The model under review builds one solid part; all positions refer to its coordinate system, in mm. Face numbers are marked on the shaded views. Give positions to 0.01 mm unless a question says otherwise; leave off trailing zeros. Order: outer loops, then holes, each group sorted by start corner. A loop starts at its lowest first (then second) coordinate and runs counter-clockwise, first axis right, second up. Notation, with made-up numbers: (-2.75, -8) - (4.25, -8) arc R31 cw to (4.25, 20) - close; hole circle Ø5 at (75.25, -6.5). An arc over 180 degrees is marked (long way). Put each result on its own line as item: value.
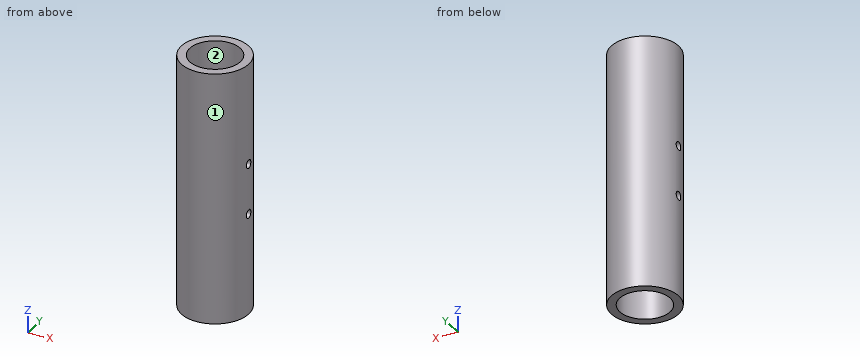
```python
from build123d import *

# Parameters (mm, degrees)
SKETCH1_R               = 20
BOSS_EXTRUDE1_DEPTH     = 150
SKETCH2_R               = 15
CUT_EXTRUDE1_DEPTH      = 150
CUT_EXTRUDE2_DEPTH      = 153.643375225
CUT_EXTRUDE2_DEPTH_BACK = 153.643375225
SKETCH3_R               = 2.5


with BuildPart() as part:
    # Sketch1 → Boss-Extrude1 (new body)
    with BuildSketch(Plane.XY):
        Circle(SKETCH1_R)
    extrude(amount=BOSS_EXTRUDE1_DEPTH)

    # Sketch2 → Cut-Extrude1 (cut)
    with BuildSketch(Plane.XY.offset(150)):
        Circle(SKETCH2_R)
    extrude(amount=-CUT_EXTRUDE1_DEPTH, mode=Mode.SUBTRACT)

    # Sketch3 → Cut-Extrude2 (cut, two sides: drawn at the far end of the back side and taken through both)
    with BuildSketch(Plane(origin=(0, 0, 0), x_dir=(0, 0, -1), z_dir=(1, 0, 0)).offset(-CUT_EXTRUDE2_DEPTH_BACK)):
        with Locations((-90, 0)):
            Circle(SKETCH3_R)
        with Locations((-60.081308212, 0)):
            Circle(SKETCH3_R)
    extrude(amount=CUT_EXTRUDE2_DEPTH + CUT_EXTRUDE2_DEPTH_BACK, mode=Mode.SUBTRACT)


solid = part.part
```
(1) The part is to be moulded in two halves that separate along Y. For the marked faces 1 and 2, say which applies: pulls with the +Y half, pulls with the -Y half, needs draft (parallel to the pull), parting line crosses it, or undercut.
The answers:
face 1: parting line crosses it
face 2: undercut
(2) Clearance check with flat-ended pins moving along their axes: pin 1 Ø12 at (y, z) = (11.5, 105) entering from +X; pin 2 Ø1.5 at (x, z) = (-9, 75) entering from -Y; pin 3 Ø12 at (x, z) = (15, 113.5) entering from -Y; pin 4 Ø4.5 at (y, z) = (0, 60.08) entering from +X. State where each tip first meets the part, or that it passes through.
The answers:
pin 1: x = 19.23
pin 2: y = -18.22
pin 3: y = -17.86
pin 4: through
(3) Take a section at C-C, the plane y = 0. Write out the cut boundary in (x, z), then the cut area to 3 significant figures.
The answers:
outline: (-20, 0) - (-15, 0) - (-15, 57.58) - (-20, 57.58) - close; (-20, 62.58) - (-15, 62.58) - (-15, 87.5) - (-20, 87.5) - close; (-20, 92.5) - (-15, 92.5) - (-15, 150) - (-20, 150) - close; (15, 0) - (20, 0) - (20, 57.58) - (15, 57.58) - close; (15, 62.58) - (20, 62.58) - (20, 87.5) - (15, 87.5) - close; (15, 92.5) - (20, 92.5) - (20, 150) - (15, 150) - close
area: 1,400 mm^2
(4) Take a section at A-A, the plane x = 0. Write out the cut boundary in (y, z).
The answers:
outline: (-20, 0) - (-15, 0) - (-15, 150) - (-20, 150) - close; (15, 0) - (20, 0) - (20, 150) - (15, 150) - close
(5) Take a section at B-B, the plane y = -9.5. Write out the cut boundary in (x, z).
The answers:
outline: (-17.6, 0) - (-11.61, 0) - (-11.61, 150) - (-17.6, 150) - close; (11.61, 0) - (17.6, 0) - (17.6, 150) - (11.61, 150) - close
(6) Take a section at D-D, the plane z = 49.5. Write out the cut boundary in (x, y), then the cut area to 3 significant figures.
The answers:
outline: circle Ø40 at (0, 0); hole circle Ø30 at (0, 0)
area: 550 mm^2
(7) Wall thickness on L1, parallel to Z at x = 16.5, y = 0; L2, parallel to Y at x = 0, z = 94; L3, parallel to Y at x = -10.5, z = 110: over which ranges is each line inside the solid? List them lowest first.
The answers:
L1: 0 to 57.58, 62.58 to 87.5, 92.5 to 150
L2: -20 to -15, 15 to 20
L3: -17.02 to -10.71, 10.71 to 17.02
